Build history of the part. All positions in model axes, mm. Face numbers are marked on the shaded views. A direction names the side the tool comes from. Round coordinates to 2 decimals unless told otherwise and drop trailing zeros. Write each loop counter-clockwise with the first axis right and the second up, starting at its lowest first coordinate (ties: lowest second). Pieces come first, ordered by that corner, then holes. Notation, with made-up numbers: (66.5, 82.5) -> (76.5, 82.5) arc R25 cw to (76.5, 96.5) -> close; hole circle Ø8 at (-38.5, 57.25). An arc over 180 degrees is marked (long way). Answer as CSV lines item,"result".
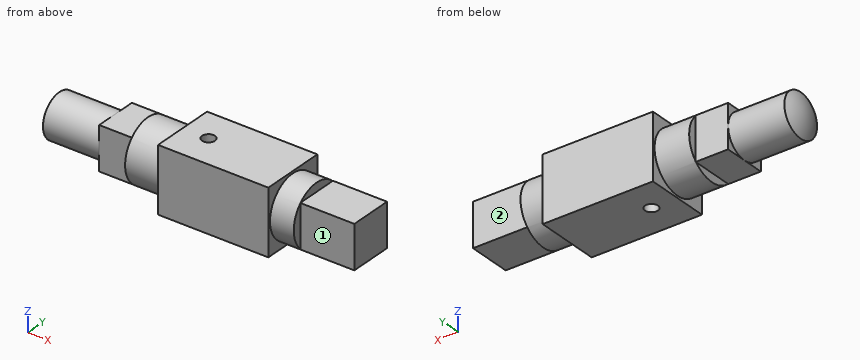
from build123d import *
from build123d.topology import SkipClean

# Parameters (mm, degrees)
SCHIZZO1_W                    = 15
SCHIZZO1_H                    = 15
ESTRUSIONE_ESTRUSIONE1_DEPTH  = 72
SCHIZZO2_W                    = 15
SCHIZZO2_H                    = 15
SCHIZZO2_R                    = 5
TAGLIO_ESTRUSIONE1_DEPTH      = 13
SCHIZZO3_W                    = 15
SCHIZZO3_H                    = 15
SCHIZZO3_W_2                  = 10
SCHIZZO3_H_2                  = 10
TAGLIO_ESTRUSIONE2_DEPTH      = 7.5
SCHIZZO4_W                    = 15
SCHIZZO4_H                    = 15
SCHIZZO4_R                    = 7
TAGLIO_ESTRUSIONE3_DEPTH      = 8
SCHIZZO6_W                    = 15
SCHIZZO6_H                    = 15
SCHIZZO6_W_2                  = 10
SCHIZZO6_H_2                  = 10
TAGLIO_ESTRUSIONE4_DEPTH      = 12.5
TAGLIO_ESTRUSIONE5_START      = -5.5
SCHIZZO8_W                    = 15
SCHIZZO8_H                    = 15
SCHIZZO8_R                    = 7
TAGLIO_ESTRUSIONE5_DEPTH      = 5.5
TAGLIO_ESTRUSIONE6_DEPTH      = 73.777056824
TAGLIO_ESTRUSIONE6_DEPTH_BACK = 73.777056824
SCHIZZO9_R                    = 1.5


with BuildPart() as part:
    # Schizzo1 → Estrusione-Estrusione1 (new body)
    with BuildSketch(Plane(origin=(0, 0, 0), x_dir=(0, 0, -1), z_dir=(1, 0, 0))):
        Rectangle(SCHIZZO1_W, SCHIZZO1_H)
    extrude(amount=ESTRUSIONE_ESTRUSIONE1_DEPTH)

    # Schizzo2 → Taglio-Estrusione1 (cut)
    with BuildSketch(Plane.ZY):
        Rectangle(SCHIZZO2_W, SCHIZZO2_H)
        Circle(SCHIZZO2_R, mode=Mode.SUBTRACT)
    extrude(amount=-TAGLIO_ESTRUSIONE1_DEPTH, mode=Mode.SUBTRACT)

    # Schizzo3 → Taglio-Estrusione2 (cut)
    with BuildSketch(Plane.ZY.offset(-13)):
        Rectangle(SCHIZZO3_W, SCHIZZO3_H)
        Rectangle(SCHIZZO3_W_2, SCHIZZO3_H_2, mode=Mode.SUBTRACT)
    extrude(amount=-TAGLIO_ESTRUSIONE2_DEPTH, mode=Mode.SUBTRACT)

    # Schizzo4 → Taglio-Estrusione3 (cut)
    with BuildSketch(Plane.ZY.offset(-20.5)):
        Rectangle(SCHIZZO4_W, SCHIZZO4_H)
        Circle(SCHIZZO4_R, mode=Mode.SUBTRACT)
    extrude(amount=-TAGLIO_ESTRUSIONE3_DEPTH, mode=Mode.SUBTRACT)

    # Schizzo5 → Rivoluzione1 (revolve)
    with SkipClean():  # the faces are left unmerged after this step: merging them gives an invalid solid
        with BuildSketch(Plane.XY):
            with BuildLine():
                Line((0, 0), (0, 5.008991915))
                ThreePointArc((0, 5.008991915), (-0.969704108, 2.587469807), (-1.3, 0))
                Line((-1.3, 0), (0, 0))
            make_face()
            with BuildLine():
                Line((0, -5.008991915), (0, 0))
                Line((0, 0), (-1.3, 0))
                ThreePointArc((-1.3, 0), (-0.969704108, -2.587469807), (0, -5.008991915))
            make_face()
        revolve(axis=Axis((0, 0, 0), (-1, 0, 0)))
    add(part.part.scale(1), mode=Mode.REPLACE)  # the faces are merged on a copy

    # Schizzo6 → Taglio-Estrusione4 (cut)
    with BuildSketch(Plane(origin=(72, 0, 0), x_dir=(0, 0, -1), z_dir=(1, 0, 0))):
        Rectangle(SCHIZZO6_W, SCHIZZO6_H)
        Rectangle(SCHIZZO6_W_2, SCHIZZO6_H_2, mode=Mode.SUBTRACT)
    extrude(amount=-TAGLIO_ESTRUSIONE4_DEPTH, mode=Mode.SUBTRACT)

    # Schizzo8 → Taglio-Estrusione5 (cut)
    with BuildSketch(Plane(origin=(59.5, 0, 0), x_dir=(0, 0, -1), z_dir=(1, 0, 0)).offset(TAGLIO_ESTRUSIONE5_START)):
        Rectangle(SCHIZZO8_W, SCHIZZO8_H)
        with Locations(Location((0, 0, 0), (0, 0, 180))):
            Circle(SCHIZZO8_R, mode=Mode.SUBTRACT)
    extrude(amount=TAGLIO_ESTRUSIONE5_DEPTH, mode=Mode.SUBTRACT)

    # Schizzo9 → Taglio-Estrusione6 (cut, two sides: drawn at the far end of the back side and taken through both)
    with BuildSketch(Plane.XY.offset(-TAGLIO_ESTRUSIONE6_DEPTH_BACK)):
        with Locations((34.5, 0)):
            Circle(SCHIZZO9_R)
    extrude(amount=TAGLIO_ESTRUSIONE6_DEPTH + TAGLIO_ESTRUSIONE6_DEPTH_BACK, mode=Mode.SUBTRACT)


solid = part.part
1. Probe line 1 along X through (y, z) = (0, 0.5); line 2 along Y through (x, z) = (34.5, 0.5); line 3 along Z through (x, y) = (63.5, -3.5). List the from-to ranges inside material, lowest first.
Results found:
line 1,"x = -1.29 to 33, 36 to 72"
line 2,"y = -7.5 to -1.5, 1.5 to 7.5"
line 3,"z = -5 to 5"
2. Cut at A-A, the plane x = 34.5. Write the cut outline in (y, z), then the cut area to 3 significant figures.
Results found:
outline,"(-7.5, -7.5) -> (-1.5, -7.5) -> (-1.5, 7.5) -> (-7.5, 7.5) -> close; (1.5, -7.5) -> (7.5, -7.5) -> (7.5, 7.5) -> (1.5, 7.5) -> close"
area,"180 mm2"
3. Cut at D-D, the plane x = 65.5. Write the cut outline in (y, z), then the cut area to 3 significant figures.
Results found:
outline,"(-5, -5) -> (5, -5) -> (5, 5) -> (-5, 5) -> close"
area,"100 mm2"
4. Drop flat-ended pins along their axis: pin 1 Ø6 at (x, y) = (18.5, 0) entering from -Z; pin 2 Ø1 at (y, z) = (-3.5, -0.5) entering from -X; pin 3 Ø1 at (y, z) = (6, 0.5) entering from -X. Give the stop position or say it passes through.
Results found:
pin 1,"stops at z = -7"
pin 2,"stops at x = -0.84"
pin 3,"stops at x = 20.5"
5. Which spindle directions (+Z, -Z, +X, -X, +Y, -Y) get a long thin tool onto all of the face, cutting with end or side? Do the marked faces 1 and 2. Say none if no direction does.
Results found:
face 1,"+Z, -Z, +X, -Y"
face 2,"+Z, -Z, +X, +Y"
